```python
from build123d import *

# Parameters (mm, degrees)
BOSS_EXTRUDE1_DEPTH      = 30.734
SKETCH2_R                = 3.302
CUT_EXTRUDE3_DEPTH       = 45.196
FILLET3_R                = 5.08
FILLET4_R                = 2.54
SKETCH3_R                = 5.08
CUT_EXTRUDE5_DEPTH       = 41.64
CUT_EXTRUDE5_DEPTH_BACK  = 1
CUT_EXTRUDE14_DEPTH      = 41.64
CUT_EXTRUDE14_DEPTH_BACK = 1


with BuildPart() as part:
    # Sketch1 → Boss-Extrude1 (new body)
    with BuildSketch(Plane.XY):
        Polygon((0, 0), (40.64, 0), (40.64, 44.196), (37.147341265, 44.196), (37.147341265, 4.043206852), (4.107237524, 4.043206852), (4.107237524, 44.196), (0, 44.196), align=None)
    extrude(amount=BOSS_EXTRUDE1_DEPTH)

    # Sketch2 → Cut-Extrude3 (cut, through all)
    with BuildSketch(Plane.XZ):
        with Locations(Location((20.066, 10.414, 0), (0, 0, 270))):  # turned: the seam where the file's is
            Circle(SKETCH2_R)
        with BuildLine():
            Line((16.764, 30.734), (23.368, 30.734))
            Line((23.368, 30.734), (23.368, 25.146))
            ThreePointArc((23.368, 25.146), (20.066, 21.844), (16.764, 25.146))
            Line((16.764, 25.146), (16.764, 30.734))
        make_face()
    extrude(amount=-CUT_EXTRUDE3_DEPTH, mode=Mode.SUBTRACT)

    # Fillet3
    fillet3_edges = [part.edges().sort_by_distance(p)[0] for p in [
        (40.64, 0, 15.367),
        (0, 0, 15.367),
    ]]
    fillet(fillet3_edges, radius=FILLET3_R)

    # Fillet4
    fillet4_edges = [part.edges().sort_by_distance(p)[0] for p in [
        (4.107237524, 4.043206852, 15.367),
        (37.147341265, 4.043206852, 15.367),
    ]]
    fillet(fillet4_edges, radius=FILLET4_R)

    # Sketch3 → Cut-Extrude5 (cut, two sides)
    with BuildSketch(Plane(origin=(0, 0, 0), x_dir=(0, 0, -1), z_dir=(1, 0, 0))) as cut_extrude5_sk:
        with Locations((-21.717, 35.179)):
            Circle(SKETCH3_R)
    extrude(amount=CUT_EXTRUDE5_DEPTH, mode=Mode.SUBTRACT)
    extrude(cut_extrude5_sk.sketch, amount=-CUT_EXTRUDE5_DEPTH_BACK, mode=Mode.SUBTRACT)

    # Sketch6 → Cut-Extrude14 (cut, two sides)
    with BuildSketch(Plane(origin=(0, 0, 0), x_dir=(0, 0, -1), z_dir=(1, 0, 0))) as cut_extrude14_sk:
        with BuildLine():
            Line((-30.734, 44.196), (-30.734, 35.179))
            ThreePointArc((-30.734, 35.179), (-28.092981846, 41.554981846), (-21.717, 44.196))
            Line((-21.717, 44.196), (-30.734, 44.196))
        make_face()
        with BuildLine():
            Line((0, 44.196), (-21.717, 44.196))
            ThreePointArc((-21.717, 44.196), (-17.535826364, 43.167997185), (-14.308020426, 40.318388162))
            Line((-14.308020426, 40.318388162), (-1.524, 21.888850787))
            ThreePointArc((-1.524, 21.888850787), (-0.389894225, 19.569850475), (0, 17.018))
            Line((0, 17.018), (0, 44.196))
        make_face()
    extrude(amount=CUT_EXTRUDE14_DEPTH, mode=Mode.SUBTRACT)
    extrude(cut_extrude14_sk.sketch, amount=-CUT_EXTRUDE14_DEPTH_BACK, mode=Mode.SUBTRACT)


solid = part.part
```
The model under review builds one solid part; all positions refer to its coordinate system, in mm. A direction names the side the tool comes from. Round coordinates to 2 decimals unless told otherwise and drop trailing zeros. Order: outer loops, then holes, each group sorted by start corner. A loop starts at its lowest first (then second) coordinate and runs counter-clockwise, first axis right, second up.
Item 1: Add section B-B, the plane z = 26. State the section outline as (x, y) points, and give its area (3 significant figures).
Working result:
outline: (0, 5.08) arc R5.08 ccw to (5.08, 0) - (16.76, 0) - (16.76, 4.04) - (6.65, 4.04) arc R2.54 cw to (4.11, 6.58) - (4.11, 32.45) - (0, 32.45) - close; (0, 37.91) - (4.11, 37.91) - (4.11, 43.11) - (0, 43.11) - close; (23.37, 0) - (35.56, 0) arc R5.08 ccw to (40.64, 5.08) - (40.64, 32.45) - (37.15, 32.45) - (37.15, 6.58) arc R2.54 cw to (34.61, 4.04) - (23.37, 4.04) - close; (37.15, 37.91) - (40.64, 37.91) - (40.64, 43.11) - (37.15, 43.11) - close
area: 385 mm2
Item 2: For pin 1 (6 mm diameter, centred on y = 30.5, z = 7, fed in from +X); pin 2 (2 mm diameter, centred on y = 1.5, z = 27.5, fed in from +X); pin 3 (3 mm diameter, centred on x = 7, z = 14, fed in from +Y); pin 4 (1.2 mm diameter, centred on y = 1.5, z = 29, fed in from -X), all flat-tipped, find the tip position at first contact; note any pin that passes through.
Working result:
pin 1: stops at x = 40.64
pin 2: stops at x = 39.94
pin 3: stops at y = 4.32
pin 4: stops at x = 0.97
Item 3: Add section D-D, the plane y = 27. State the section outline as (x, z) points.
Working result:
outline: (0, 5.07) - (4.11, 5.07) - (4.11, 30.73) - (0, 30.73) - close; (37.15, 5.07) - (40.64, 5.07) - (40.64, 30.73) - (37.15, 30.73) - close
Item 4: Machinability: for faces 1 (the flat face through (3, 14, 30.734)), 2 (the cylindrical face through (4.83, 4.81, 15.58)), 3 (the flat face through (16.764, 2, 28)), which of the approach directions +Z, -Z, +X, -X, +Y, -Y give a long, thin tool a straight path to every point of the face, cutting with its end or side? Answer none if there is none.
Working result:
face 1: +Z, +X, -X, +Y, -Y
face 2: +Z, -Z, +Y
face 3: +Z, +Y, -Y
Item 5: To check wall thickness, follow probe 1 along X at (y, z) = (36, 28.5); probe 2 along Y at (x, z) = (9.5, 17); probe 3 along X at (y, z) = (3, 10). State the ranges of each line that lie inside material, in increasing order.
Working result:
probe 1: x = 0 to 4.11, 37.15 to 40.64
probe 2: y = 0 to 4.04
probe 3: x = 0.45 to 16.79, 23.34 to 40.19
Item 6: Draft analysis for pull direction Z (two halves, no side actions). For faces 4 (the flat face through (20, 3, 0)), 5 (the flat face through (37.147, 21, 15)), 6 (the cylindrical face through (38.869, 38.612, 25.461)), state which applies: released by +Z, released by -Z, zero draft, split by the parting line, or undercut.
Working result:
face 4: released by -Z
face 5: zero draft
face 6: undercut
Item 7: Add section C-C, the plane z = 20. State the section outline as (x, y) points, and give its area (3 significant figures).
Working result:
outline: (0, 5.08) arc R5.08 ccw to (5.08, 0) - (35.56, 0) arc R5.08 ccw to (40.64, 5.08) - (40.64, 30.4) - (37.15, 30.4) - (37.15, 6.58) arc R2.54 cw to (34.61, 4.04) - (6.65, 4.04) arc R2.54 cw to (4.11, 6.58) - (4.11, 30.4) - (0, 30.4) - close; (0, 39.96) - (4.11, 39.96) - (4.11, 44.03) - (0, 44.03) - close; (37.15, 39.96) - (40.64, 39.96) - (40.64, 44.03) - (37.15, 44.03) - close
area: 387 mm2
Item 8: Add section A-A, the plane y = 13. State the section outline as (x, z) points, and give its area (3 significant figures).
Working result:
outline: (0, 0) - (4.11, 0) - (4.11, 30.73) - (0, 30.73) - close; (37.15, 0) - (40.64, 0) - (40.64, 30.73) - (37.15, 30.73) - close
area: 234 mm2
